The listing builds one solid part. Answer for the finished solid, in the listing's coordinates (mm). Coordinates: 2 decimals unless noted, no trailing zeros. Write each loop counter-clockwise with the first axis right and the second up, starting at its lowest first coordinate (ties: lowest second). Pieces come first, ordered by that corner, then holes. Notation, with made-up numbers: M -33.75,42 L -25.75,42 A24 ccw -25.75,62 Z; hole C -21,-8.5 d4. An arc over 180 degrees is marked long. Write item = value, one per line. Start each with the question number.
```python
from build123d import *

# Parameters (mm, degrees)
SKETCH1_W           = 100
SKETCH1_H           = 160
BOSS_EXTRUDE1_DEPTH = 12.7
SKETCH2_R           = 4.5
CUT_EXTRUDE1_DEPTH  = 12.7
SKETCH3_R           = 4.5
CUT_EXTRUDE2_DEPTH  = 12.7


with BuildPart() as part:
    # Sketch1 → Boss-Extrude1 (new body)
    with BuildSketch(Plane.XY):
        with Locations((50, 80)):
            Rectangle(SKETCH1_W, SKETCH1_H)
    extrude(amount=BOSS_EXTRUDE1_DEPTH)

    # Sketch2 → Cut-Extrude1 (cut)
    with BuildSketch(Plane(origin=(0, 0, 12.7), x_dir=(-1, 0, 0), z_dir=(0, 0, 1))):
        with Locations(Location((-75, -110, 0), (0, 0, 180))):
            Circle(SKETCH2_R)
        with Locations(Location((-25, -110, 0), (0, 0, 180))):
            Circle(SKETCH2_R)
        with Locations((-25, -50)):
            Circle(SKETCH2_R)
        with Locations((-75, -50)):
            Circle(SKETCH2_R)
    extrude(amount=-CUT_EXTRUDE1_DEPTH, mode=Mode.SUBTRACT)

    # Sketch3 → Cut-Extrude2 (cut)
    with BuildSketch(Plane.XY.offset(12.7)):
        with Locations((14, 15)):
            Circle(SKETCH3_R)
        with Locations((86, 15)):
            Circle(SKETCH3_R)
        with Locations(Location((14, 145, 0), (0, 0, 180))):
            Circle(SKETCH3_R)
        with Locations(Location((86, 145, 0), (0, 0, 180))):
            Circle(SKETCH3_R)
    extrude(amount=-CUT_EXTRUDE2_DEPTH, mode=Mode.SUBTRACT)


solid = part.part
```
1. Straight lines are drawn through the part: L1, parallel to Y at x = 75, z = 4; L2, parallel to Y at x = 14, z = 1.75; L3, parallel to X at y = 17.5, z = 9. For each, find the intervals that lie inside material, in ascending order. Write a range as [from, to].
2. The part is cut by section C-C, the plane z = 3.5. Count the separate pieces of the cut face and the enclosed holes in it, and give its area (3 significant figures).
3. For a pull along Y with two mould halves and no side action, classify faces 1 (the face through (81.504, 15.198, 6.439)), 2 (the face through (49, 0, 6)), 3 (the face through (49, 160, 6)), 4 (the face through (49, 81, 12.7)) as pulls with the +Y half, pulls with the -Y half, needs draft (parallel to the pull), parting line crosses it, or undercut.
4. The part is cut by section B-B, the plane x = 75. Write down the section's boundary in (y, z).
5. The part is cut by section A-A, the plane y = 15. Write down the section's boundary in (x, z), and give its area (3 significant figures).
Solution:
q1.L1 = [0, 45.5], [54.5, 105.5], [114.5, 160]
q1.L2 = [0, 10.5], [19.5, 140.5], [149.5, 160]
q1.L3 = [0, 10.26], [17.74, 82.26], [89.74, 100]
q2.separate_pieces = 1
q2.enclosed_holes = 8
q2.area = 15,500 mm^2
q3.face_1 = undercut
q3.face_2 = pulls with the -Y half
q3.face_3 = pulls with the +Y half
q3.face_4 = needs draft
q4.outline = M 0,0 L 45.5,0 L 45.5,12.7 L 0,12.7 Z; M 54.5,0 L 105.5,0 L 105.5,12.7 L 54.5,12.7 Z; M 114.5,0 L 160,0 L 160,12.7 L 114.5,12.7 Z
q5.outline = M 0,0 L 9.5,0 L 9.5,12.7 L 0,12.7 Z; M 18.5,0 L 81.5,0 L 81.5,12.7 L 18.5,12.7 Z; M 90.5,0 L 100,0 L 100,12.7 L 90.5,12.7 Z
q5.area = 1,040 mm^2
